Check sheet for the modelled part. Datum: model origin and axes. Units: mm. A direction names the side the tool comes from. Round coordinates to 2 decimals unless told otherwise and drop trailing zeros. Loops run counter-clockwise (first coordinate to the right, second up) from the corner with the lowest first, then second, coordinate; pieces in that order, holes last. Notation, with made-up numbers: M 25.25,27 L 71.25,27 A28 ccw 71.25,51 Z; hole C 75,67 d9. An arc over 180 degrees is marked long. One line per question, with ' | ' between items. Start each with the question number.
(1) Thickness scan on probe 1 along Y at (x, z) = (-1533, 188.5); probe 2 along Y at (x, z) = (-1532.5, -7.5); probe 3 along Y at (x, z) = (-1513.5, -51.5). Record the ranges inside material, lowest first. Write a range as [from, to].
(2) Go/stop test with flat-tipped pins: P1, Ø4.5, axis at x = -1513.27, y = 3555.78, coming from the -Z side; P2, Ø2.5, axis at y = 3553, z = 56.5, coming from the +X side; P3, Ø1, axis at y = 3567.5, z = 159.5, coming from the +X side (3 decimals); P4, Ø2, axis at x = -1524.5, z = 146.5, coming from the +Y side. Record where each tip stops, or that it passes through.
(3) Section check B-B (z = 73.5). Count the separate pieces of the cut face and the enclosed holes in it, and give its area (3 significant figures).
(4) Draft check along X on faces 3 (the face through (-1508.295, 3581, 52)), 4 (the face through (-1518.245, 3556, 52)), 5 (the face through (-1518, 3550.804, 52)). Enter one of: +X half, -X half, draft (parallel to the pull), parting line (faces both ways), or undercut.
(5) Section check A-A (x = -1527.5). Record the boundary of the cut face in (y, z).
(6) Tool access check on faces 1 (the face through (-1539, 3550.804, 52)), 2 (the face through (-1543, 3560.754, 52)). Record the directions out of +Z, -Z, +X, -X, +Y, -Y that give a thin tool (end or side, any length) a straight path to the whole face; none if there is none.
```python
from build123d import *

# Parameters (mm, degrees)
SKETCH_1_R      = 2.95
SKETCH_1_R_2    = 3.4
EXTRUDE_1_DEPTH = 160


with BuildPart() as part:
    # 草图1 → 凸台-拉伸1 (new body, symmetric)
    with BuildSketch(Plane.XY.offset(50)):
        with BuildLine():
            Line((-1518.245004392, 3588.004280474), (-1518.245004392, 3582.975600817))
            Line((-1518.245004392, 3582.975600817), (-1522.916324736, 3578.304280474))
            Line((-1522.916324736, 3578.304280474), (-1533.673684048, 3578.304280474))
            Line((-1533.673684048, 3578.304280474), (-1538.345004392, 3582.975600817))
            Line((-1538.345004392, 3582.975600817), (-1538.345004392, 3588.004280474))
            Line((-1538.345004392, 3588.004280474), (-1534.845004392, 3588.004280474))
            Line((-1534.845004392, 3588.004280474), (-1534.845004392, 3586.304280474))
            Line((-1534.845004392, 3586.304280474), (-1532.445004392, 3586.304280474))
            Line((-1532.445004392, 3586.304280474), (-1532.445004392, 3589.704280474))
            ThreePointArc((-1532.445004392, 3589.704280474), (-1532.503583036, 3589.84570183), (-1532.645004392, 3589.904280474))
            Line((-1532.645004392, 3589.904280474), (-1533.345004392, 3589.904280474))
            Line((-1533.345004392, 3589.904280474), (-1533.345004392, 3590.604280474))
            ThreePointArc((-1533.345004392, 3590.604280474), (-1533.403583036, 3590.74570183), (-1533.545004392, 3590.804280474))
            Line((-1533.545004392, 3590.804280474), (-1543.795004392, 3590.804280474))
            ThreePointArc((-1543.795004392, 3590.804280474), (-1546.976984907, 3589.486260989), (-1548.295004392, 3586.304280474))
            Line((-1548.295004392, 3586.304280474), (-1548.295004392, 3576.054280474))
            ThreePointArc((-1548.295004392, 3576.054280474), (-1548.236425748, 3575.912859117), (-1548.095004392, 3575.854280474))
            Line((-1548.095004392, 3575.854280474), (-1547.395004392, 3575.854280474))
            Line((-1547.395004392, 3575.854280474), (-1547.395004392, 3575.154280474))
            ThreePointArc((-1547.395004392, 3575.154280474), (-1547.336425748, 3575.012859117), (-1547.195004392, 3574.954280474))
            Line((-1547.195004392, 3574.954280474), (-1543.795004392, 3574.954280474))
            Line((-1543.795004392, 3574.954280474), (-1543.795004392, 3577.354280474))
            Line((-1543.795004392, 3577.354280474), (-1545.495004392, 3577.354280474))
            Line((-1545.495004392, 3577.354280474), (-1545.495004392, 3580.854280474))
            Line((-1545.495004392, 3580.854280474), (-1540.466324736, 3580.854280474))
            Line((-1540.466324736, 3580.854280474), (-1535.795004392, 3576.18296013))
            Line((-1535.795004392, 3576.18296013), (-1535.795004392, 3565.425600817))
            Line((-1535.795004392, 3565.425600817), (-1540.466324736, 3560.754280474))
            Line((-1540.466324736, 3560.754280474), (-1545.495004392, 3560.754280474))
            Line((-1545.495004392, 3560.754280474), (-1545.495004392, 3564.254280474))
            Line((-1545.495004392, 3564.254280474), (-1543.795004392, 3564.254280474))
            Line((-1543.795004392, 3564.254280474), (-1543.795004392, 3566.654280474))
            Line((-1543.795004392, 3566.654280474), (-1547.195004392, 3566.654280474))
            ThreePointArc((-1547.195004392, 3566.654280474), (-1547.336425748, 3566.59570183), (-1547.395004392, 3566.454280474))
            Line((-1547.395004392, 3566.454280474), (-1547.395004392, 3565.754280474))
            Line((-1547.395004392, 3565.754280474), (-1548.095004392, 3565.754280474))
            ThreePointArc((-1548.095004392, 3565.754280474), (-1548.236425748, 3565.69570183), (-1548.295004392, 3565.554280474))
            Line((-1548.295004392, 3565.554280474), (-1548.295004392, 3555.304280474))
            ThreePointArc((-1548.295004392, 3555.304280474), (-1546.976984907, 3552.122299958), (-1543.795004392, 3550.804280474))
            Line((-1543.795004392, 3550.804280474), (-1533.545004392, 3550.804280474))
            ThreePointArc((-1533.545004392, 3550.804280474), (-1533.403583036, 3550.862859117), (-1533.345004392, 3551.004280474))
            Line((-1533.345004392, 3551.004280474), (-1533.345004392, 3551.704280474))
            Line((-1533.345004392, 3551.704280474), (-1532.645004392, 3551.704280474))
            ThreePointArc((-1532.645004392, 3551.704280474), (-1532.503583036, 3551.762859117), (-1532.445004392, 3551.904280474))
            Line((-1532.445004392, 3551.904280474), (-1532.445004392, 3555.304280474))
            Line((-1532.445004392, 3555.304280474), (-1534.845004392, 3555.304280474))
            Line((-1534.845004392, 3555.304280474), (-1534.845004392, 3553.604280474))
            Line((-1534.845004392, 3553.604280474), (-1538.345004392, 3553.604280474))
            Line((-1538.345004392, 3553.604280474), (-1538.345004392, 3558.63296013))
            Line((-1538.345004392, 3558.63296013), (-1533.673684048, 3563.304280474))
            Line((-1533.673684048, 3563.304280474), (-1522.916324736, 3563.304280474))
            Line((-1522.916324736, 3563.304280474), (-1518.245004392, 3558.63296013))
            Line((-1518.245004392, 3558.63296013), (-1518.245004392, 3553.604280474))
            Line((-1518.245004392, 3553.604280474), (-1521.745004392, 3553.604280474))
            Line((-1521.745004392, 3553.604280474), (-1521.745004392, 3555.304280474))
            Line((-1521.745004392, 3555.304280474), (-1524.145004392, 3555.304280474))
            Line((-1524.145004392, 3555.304280474), (-1524.145004392, 3551.904280474))
            ThreePointArc((-1524.145004392, 3551.904280474), (-1524.086425748, 3551.762859117), (-1523.945004392, 3551.704280474))
            Line((-1523.945004392, 3551.704280474), (-1523.245004392, 3551.704280474))
            Line((-1523.245004392, 3551.704280474), (-1523.245004392, 3551.004280474))
            ThreePointArc((-1523.245004392, 3551.004280474), (-1523.186425748, 3550.862859117), (-1523.045004392, 3550.804280474))
            Line((-1523.045004392, 3550.804280474), (-1512.795004392, 3550.804280474))
            ThreePointArc((-1512.795004392, 3550.804280474), (-1509.613023877, 3552.122299958), (-1508.295004392, 3555.304280474))
            Line((-1508.295004392, 3555.304280474), (-1508.295004392, 3565.554280474))
            ThreePointArc((-1508.295004392, 3565.554280474), (-1508.353583036, 3565.69570183), (-1508.495004392, 3565.754280474))
            Line((-1508.495004392, 3565.754280474), (-1509.195004392, 3565.754280474))
            Line((-1509.195004392, 3565.754280474), (-1509.195004392, 3566.454280474))
            ThreePointArc((-1509.195004392, 3566.454280474), (-1509.253583036, 3566.59570183), (-1509.395004392, 3566.654280474))
            Line((-1509.395004392, 3566.654280474), (-1512.795004392, 3566.654280474))
            Line((-1512.795004392, 3566.654280474), (-1512.795004392, 3564.254280474))
            Line((-1512.795004392, 3564.254280474), (-1511.095004392, 3564.254280474))
            Line((-1511.095004392, 3564.254280474), (-1511.095004392, 3560.754280474))
            Line((-1511.095004392, 3560.754280474), (-1516.123684048, 3560.754280474))
            Line((-1516.123684048, 3560.754280474), (-1520.795004392, 3565.425600817))
            Line((-1520.795004392, 3565.425600817), (-1520.795004392, 3576.18296013))
            Line((-1520.795004392, 3576.18296013), (-1516.123684048, 3580.854280474))
            Line((-1516.123684048, 3580.854280474), (-1511.095004392, 3580.854280474))
            Line((-1511.095004392, 3580.854280474), (-1511.095004392, 3577.354280474))
            Line((-1511.095004392, 3577.354280474), (-1512.795004392, 3577.354280474))
            Line((-1512.795004392, 3577.354280474), (-1512.795004392, 3574.954280474))
            Line((-1512.795004392, 3574.954280474), (-1509.395004392, 3574.954280474))
            ThreePointArc((-1509.395004392, 3574.954280474), (-1509.253583036, 3575.012859117), (-1509.195004392, 3575.154280474))
            Line((-1509.195004392, 3575.154280474), (-1509.195004392, 3575.854280474))
            Line((-1509.195004392, 3575.854280474), (-1508.495004392, 3575.854280474))
            ThreePointArc((-1508.495004392, 3575.854280474), (-1508.353583036, 3575.912859117), (-1508.295004392, 3576.054280474))
            Line((-1508.295004392, 3576.054280474), (-1508.295004392, 3586.304280474))
            ThreePointArc((-1508.295004392, 3586.304280474), (-1509.613023877, 3589.486260989), (-1512.795004392, 3590.804280474))
            Line((-1512.795004392, 3590.804280474), (-1523.045004392, 3590.804280474))
            ThreePointArc((-1523.045004392, 3590.804280474), (-1523.186425748, 3590.74570183), (-1523.245004392, 3590.604280474))
            Line((-1523.245004392, 3590.604280474), (-1523.245004392, 3589.904280474))
            Line((-1523.245004392, 3589.904280474), (-1523.945004392, 3589.904280474))
            ThreePointArc((-1523.945004392, 3589.904280474), (-1524.086425748, 3589.84570183), (-1524.145004392, 3589.704280474))
            Line((-1524.145004392, 3589.704280474), (-1524.145004392, 3586.304280474))
            Line((-1524.145004392, 3586.304280474), (-1521.745004392, 3586.304280474))
            Line((-1521.745004392, 3586.304280474), (-1521.745004392, 3588.004280474))
            Line((-1521.745004392, 3588.004280474), (-1518.245004392, 3588.004280474))
        make_face()
        with Locations((-1513.270004392, 3555.779280474)):
            Circle(SKETCH_1_R, mode=Mode.SUBTRACT)
        with Locations((-1528.295004392, 3570.804280474)):
            Circle(SKETCH_1_R_2, mode=Mode.SUBTRACT)
        with Locations((-1513.270004392, 3585.829280474)):
            Circle(SKETCH_1_R, mode=Mode.SUBTRACT)
        with Locations((-1543.320004392, 3585.829280474)):
            Circle(SKETCH_1_R, mode=Mode.SUBTRACT)
        with Locations((-1543.320004392, 3555.779280474)):
            Circle(SKETCH_1_R, mode=Mode.SUBTRACT)
    extrude(amount=EXTRUDE_1_DEPTH, both=True)


solid = part.part
```
The answers:
1) probe 1: [3551.7, 3555.3], [3563.3, 3578.3], [3586.3, 3589.9] | probe 2: [3551.77, 3555.3], [3563.3, 3578.3], [3586.3, 3589.84] | probe 3: [3550.8, 3552.84], [3558.72, 3560.75], [3580.85, 3582.89], [3588.77, 3590.8]
2) P1: through | P2: x = -1508.42 | P3: x = -1520.795 | P4: y = 3589.9
3) separate pieces: 1 | enclosed holes: 5 | area: 677 mm²
4) face 3: +X half | face 4: undercut | face 5: draft
5) outline: M 3563.3,-110 L 3567.5,-110 L 3567.5,210 L 3563.3,210 Z; M 3574.11,-110 L 3578.3,-110 L 3578.3,210 L 3574.11,210 Z
6) face 1: +Z, -Z, +X, -X, -Y | face 2: +Z, -Z
